Design review of the part shown in the three views and the two pictorial views. Dimensions are in mm from the part's minimum x, y and z. A direction names the side the tool comes from. Give positions to 0.01 mm unless a question says otherwise; leave off trailing zeros. Loops run counter-clockwise (first coordinate to the right, second up) from the corner with the lowest first, then second, coordinate; pieces in that order, holes last. Notation, with made-up numbers: (10.5, 36.25) - (19.5, 36.25) arc R16 ccw to (19.5, 64.25) - close; hole circle Ø11 at (53.25, -28.5). An arc over 180 degrees is marked (long way). Answer as a JSON object with one key per item and string values.
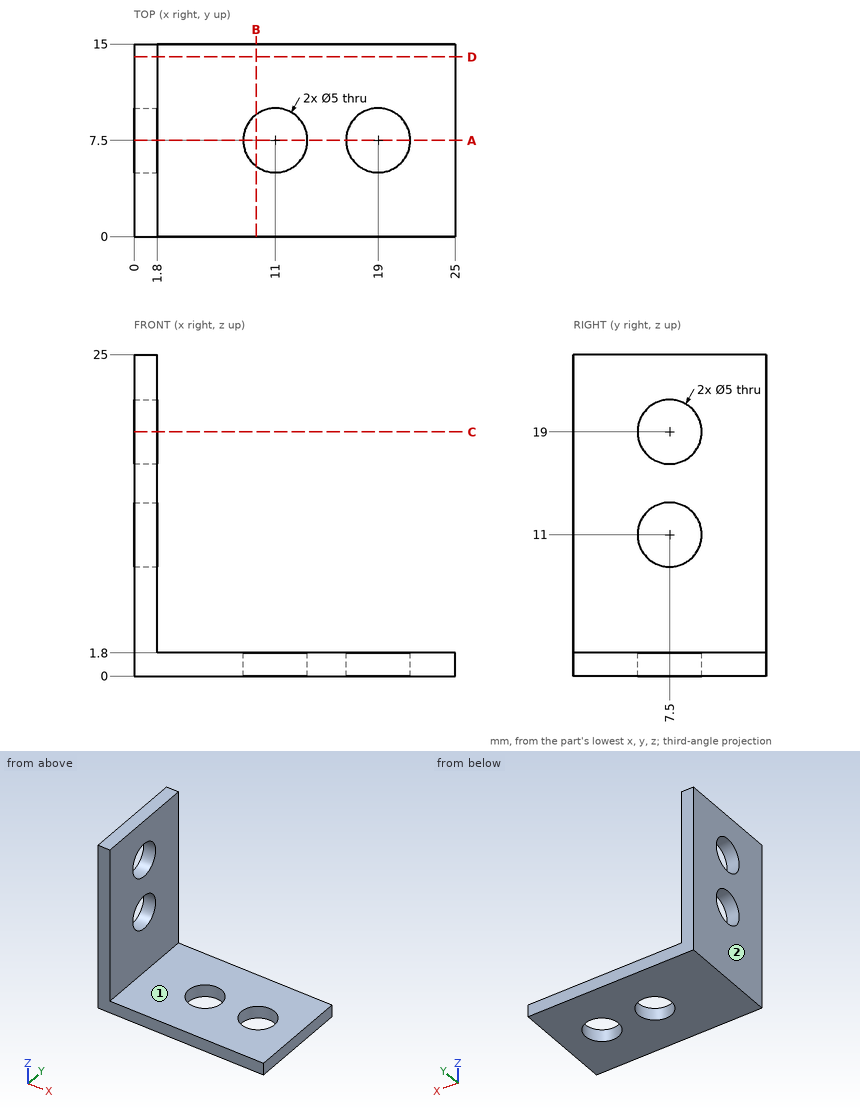
Q1. Consider section B-B, the plane x = 9.5. State the section outline as (y, z) points, plus the area to 3 significant figures.
Results:
{"outline": "(0, 0) - (5.5, 0) - (5.5, 1.8) - (0, 1.8) - close; (9.5, 0) - (15, 0) - (15, 1.8) - (9.5, 1.8) - close", "area": "19.8 mm^2"}
Q2. For the marked faces 1 and 2, list the 3-axis set-ups (+Z, -Z, +X, -X, +Y, -Y) from which the entire face can be reached by the end or side of a thin tool; tool diameter is ignored.
Results:
{"face 1": "+Z, +X, +Y, -Y", "face 2": "+Z, -Z, -X, +Y, -Y"}
Q3. Consider section A-A, the plane y = 7.5. State the section outline as (x, z) points.
Results:
{"outline": "(0, 0) - (8.5, 0) - (8.5, 1.8) - (1.8, 1.8) - (1.8, 8.5) - (0, 8.5) - close; (0, 13.5) - (1.8, 13.5) - (1.8, 16.5) - (0, 16.5) - close; (0, 21.5) - (1.8, 21.5) - (1.8, 25) - (0, 25) - close; (13.5, 0) - (16.5, 0) - (16.5, 1.8) - (13.5, 1.8) - close; (21.5, 0) - (25, 0) - (25, 1.8) - (21.5, 1.8) - close"}
Q4. Clearance check with flat-ended pins moving along their axes: pin 1 Ø4 at (y, z) = (7.5, 11) entering from +X; pin 2 Ø8 at (x, y) = (11, 7.5) entering from +Z. State where each tip first meets the part, or that it passes through.
Results:
{"pin 1": "passes through", "pin 2": "stops at z = 1.8"}
Q5. To check wall thickness, follow probe 1 along Z at (x, y) = (0.55, 7.5); probe 2 along Y at (x, z) = (0.6, 11); probe 3 along X at (y, z) = (5, 3.25). State the ranges of each line that lie inside material, in increasing order. Write a range as [from, to].
Results:
{"probe 1": "z = [0, 8.5], [13.5, 16.5], [21.5, 25]", "probe 2": "y = [0, 5], [10, 15]", "probe 3": "x = [0, 1.8]"}
Q6. Consider section C-C, the plane z = 19. State the section outline as (x, y) points.
Results:
{"outline": "(0, 0) - (1.8, 0) - (1.8, 5) - (0, 5) - close; (0, 10) - (1.8, 10) - (1.8, 15) - (0, 15) - close"}
Q7. Consider section D-D, the plane y = 14. State the section outline as (x, z) points, plus the area to 3 significant figures.
Results:
{"outline": "(0, 0) - (25, 0) - (25, 1.8) - (1.8, 1.8) - (1.8, 25) - (0, 25) - close", "area": "86.8 mm^2"}
